Geometry check sheet. Reference: the model listing, model coordinates, mm. A direction names the side the tool comes from. Round coordinates to 2 decimals unless told otherwise and drop trailing zeros. Loops run counter-clockwise (first coordinate to the right, second up) from the corner with the lowest first, then second, coordinate; pieces in that order, holes last.
```python
from build123d import *

# Parameters (mm, degrees)
SKETCH_W        = 18
SKETCH_H        = 18
PAD_DEPTH       = 6
SKETCH001_W     = 18
SKETCH001_H     = 18
SKETCH001_R     = 4.5
POCKET_DEPTH    = 3
SKETCH002_R     = 2
POCKET001_DEPTH = 6.001
CHAMFER_SIZE    = 1
FILLET_R        = 1
CHAMFER001_SIZE = 2


with BuildPart() as part:
    # Sketch → Pad (new body)
    with BuildSketch(Plane.XY):
        with Locations((9, 9)):
            Rectangle(SKETCH_W, SKETCH_H)
    extrude(amount=PAD_DEPTH)

    # Sketch001 (on Face6 of Pad) → Pocket (cut)
    with BuildSketch(Plane.XY.offset(6)):
        with Locations((9, 9)):
            Rectangle(SKETCH001_W, SKETCH001_H)
        with Locations((9, 9)):
            Circle(SKETCH001_R, mode=Mode.SUBTRACT)
    extrude(amount=-POCKET_DEPTH, mode=Mode.SUBTRACT)

    # Sketch002 (on Face8 of Pocket) → Pocket001 (cut, through all)
    with BuildSketch(Plane.XY.offset(6)):
        with Locations((9, 9)):
            Circle(SKETCH002_R)
    extrude(amount=-POCKET001_DEPTH, mode=Mode.SUBTRACT)

    # Chamfer
    chamfer_edges = [part.edges().sort_by_distance(p)[0] for p in [
        (9, 0, 3),
        (18, 9, 3),
        (9, 18, 3),
        (0, 9, 3),
    ]]
    chamfer(chamfer_edges, length=CHAMFER_SIZE)

    # Fillet
    fillet_edges = [part.edges().sort_by_distance(p)[0] for p in [
        (0, 18, 1),
        (0, 0, 1),
        (18, 18, 1),
        (18, 0, 1),
    ]]
    fillet(fillet_edges, radius=FILLET_R)

    # Chamfer001
    chamfer001_edges = [part.edges().sort_by_distance(p)[0] for p in [
        (7, 9, 0),
    ]]
    chamfer(chamfer001_edges, length=CHAMFER001_SIZE)


solid = part.part
```
1) Gauge pin test, flat ends, axial feed: pin 1 (1.5 mm diameter, centred on x = 15, z = 5, fed in from -Y); pin 2 (6.5 mm diameter, centred on x = 9, y = 9, fed in from -Z); pin 3 (1.5 mm diameter, centred on x = 8.5, z = 4.5, fed in from +Y). Record the tip position at first contact, or that the pin passes through.
Report:
pin 1: passes through
pin 2: stops at z = 0.75
pin 3: stops at y = 13.5
2) Sectioned sample at D-D, the plane z = 2.55. Record the cut outline in (x, y), then the cut area to 3 significant figures.
Report:
outline: (0.55, 0.55) - (17.45, 0.55) - (17.45, 17.45) - (0.55, 17.45) - close; hole circle Ø4 at (9, 9)
area: 273 mm2
3) Mould release check, pull along Y, two halves, no side actions. Record for faces 1 (the face through (0, 9, 1)), 2 (the face through (13.292, 10.352, 4.521)), 3 (the face through (7.526, 10.352, 4.028)): +Y half, -Y half, draft (parallel to the pull), parting line (faces both ways), or undercut.
Report:
face 1: draft
face 2: parting line
face 3: undercut
4) Access from +Z, -Z, +X, -X, +Y, -Y to the whole of each face (thin tool, end or side, straight path). Record for faces 4 (the face through (17.699, 0.285, 1.162)), 5 (the face through (12.4, 5.6, 3)).
Report:
face 4: +Z, -Z, +X, -Y
face 5: +Z
5) Scan lines: line 1 along Y through (x, z) = (9, 4.6); line 2 along Z through (x, y) = (16.5, 8); line 3 along X through (y, z) = (10.5, 4.85). Record each from-to range of solid material in increasing order.
Report:
line 1: y = 4.5 to 7, 11 to 13.5
line 2: z = 0 to 3
line 3: x = 4.76 to 7.68, 10.32 to 13.24
6) Sectioned sample at A-A, the plane y = 9. Record the cut outline in (x, z), then the cut area to 3 significant figures.
Report:
outline: (0, 0) - (5, 0) - (7, 2) - (7, 6) - (4.5, 6) - (4.5, 3) - (1, 3) - (0, 2) - close; (11, 2) - (13, 0) - (18, 0) - (18, 2) - (17, 3) - (13.5, 3) - (13.5, 6) - (11, 6) - close
area: 52.0 mm2
7) Sectioned sample at B-B, the plane z = 0.8. Record the cut outline in (x, y), then the cut area to 3 significant figures.
Report:
outline: (0, 1) arc R1 ccw to (1, 0) - (17, 0) arc R1 ccw to (18, 1) - (18, 17) arc R1 ccw to (17, 18) - (1, 18) arc R1 ccw to (0, 17) - close; hole circle Ø6.4 at (9, 9)
area: 291 mm2
